Build history of the part. All positions in model axes, mm. Face numbers are marked on the shaded views. A direction names the side the tool comes from. Round coordinates to 2 decimals unless told otherwise and drop trailing zeros. Write each loop counter-clockwise with the first axis right and the second up, starting at its lowest first coordinate (ties: lowest second). Pieces come first, ordered by that corner, then holes. Notation, with made-up numbers: (-22.5, -16) -> (18.5, -16) arc R18 cw to (18.5, 7) -> close; hole circle Ø4 at (-39, -18.75). An arc over 180 degrees is marked (long way). Answer in a Markdown table with one row per item.
```python
from build123d import *

# Parameters (mm, degrees)
BOSS_EXTRUDE1_DEPTH = 5
SKETCH2_R           = 10
BOSS_EXTRUDE2_DEPTH = 10
SKETCH3_R           = 5
CUT_EXTRUDE1_DEPTH  = 10
BOSS_EXTRUDE3_START = 10
SKETCH4_R           = 10
BOSS_EXTRUDE3_DEPTH = 10
BOSS_EXTRUDE4_DEPTH = 5
SKETCH9_R           = 5
CUT_EXTRUDE4_DEPTH  = 35


with BuildPart() as part:
    # Sketch1 → Boss-Extrude1 (new body)
    with BuildSketch(Plane.XY):
        with BuildLine():
            Line((10, 10), (10, 200))
            ThreePointArc((10, 200), (0, 210), (-10, 200))
            Line((-10, 200), (-10, 10))
            ThreePointArc((-10, 10), (0, 0), (10, 10))
        make_face()
    extrude(amount=BOSS_EXTRUDE1_DEPTH)

    # Sketch2 → Boss-Extrude2 (add)
    with BuildSketch(Plane.XY.offset(5)):
        with Locations((0, 200)):
            Circle(SKETCH2_R)
        with Locations((0, 10)):
            Circle(SKETCH2_R)
    extrude(amount=BOSS_EXTRUDE2_DEPTH)

    # Sketch3 → Cut-Extrude1 (cut)
    with BuildSketch(Plane(origin=(0, 0, 0), x_dir=(-1, 0, 0), z_dir=(0, 0, -1))):
        with Locations((0, 105)):
            Circle(SKETCH3_R)
    extrude(amount=-CUT_EXTRUDE1_DEPTH, mode=Mode.SUBTRACT)

    # Sketch4 → Boss-Extrude3 (add)
    with BuildSketch(Plane(origin=(0, 0, 0), x_dir=(-1, 0, 0), z_dir=(0, 0, -1)).offset(BOSS_EXTRUDE3_START)):
        with Locations((0, 200)):
            Circle(SKETCH4_R)
        with Locations((0, 10)):
            Circle(SKETCH4_R)
    extrude(amount=-BOSS_EXTRUDE3_DEPTH)

    # Sketch5 → Boss-Extrude4 (add)
    with BuildSketch(Plane(origin=(0, 0, 0), x_dir=(-1, 0, 0), z_dir=(0, 0, -1))):
        with BuildLine():
            Line((12, 200), (12, 10))
            ThreePointArc((12, 10), (0, -2), (-12, 10))
            Line((-12, 10), (-12, 200))
            ThreePointArc((-12, 200), (0, 212), (12, 200))
        make_face()
    extrude(amount=-BOSS_EXTRUDE4_DEPTH)

    # Sketch9 → Cut-Extrude4 (cut)
    with BuildSketch(Plane(origin=(0, 0, 0), x_dir=(-1, 0, 0), z_dir=(0, 0, -1))):
        with Locations((0, 105)):
            Circle(SKETCH9_R)
    extrude(amount=-CUT_EXTRUDE4_DEPTH, mode=Mode.SUBTRACT)


solid = part.part
```
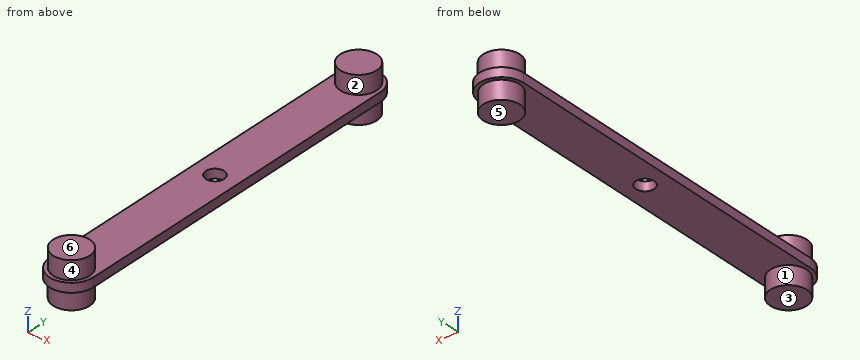
Q1. Wall check: line 1 (Y direction, x = 0, z = 1.35); line 2 (Y direction, x = 1.5, z = 6); line 3 (Z direction, x = -5.5, y = 143.5). Give the ranges that are in metal, low to high. Write a range as [from, to].
A:
| item | result |
|---|---|
| line 1 | [-2, 100], [110, 212] |
| line 2 | [0.11, 19.89], [190.11, 209.89] |
| line 3 | [0, 5] |
Q2. Saw through at A-A on x = 0. Write the cut outline in (y, z).
A:
| item | result |
|---|---|
| outline | (-2, 0) -> (0, 0) -> (0, -10) -> (20, -10) -> (20, 0) -> (100, 0) -> (100, 5) -> (20, 5) -> (20, 15) -> (0, 15) -> (0, 5) -> (-2, 5) -> close; (110, 0) -> (190, 0) -> (190, -10) -> (210, -10) -> (210, 0) -> (212, 0) -> (212, 5) -> (210, 5) -> (210, 15) -> (190, 15) -> (190, 5) -> (110, 5) -> close |
Q3. Saw through at B-B on y = 105. Write the cut outline in (x, z).
A:
| item | result |
|---|---|
| outline | (-12, 0) -> (-5, 0) -> (-5, 5) -> (-12, 5) -> close; (5, 0) -> (12, 0) -> (12, 5) -> (5, 5) -> close |
Q4. Drop flat-ended pins along their axis: P1, Ø2, axis at x = -7, z = -0.5, coming from the +Y side; P2, Ø12, axis at x = -8, z = -2.5, coming from the +Y side; P3, Ø1, axis at x = 9.5, y = 35, coming from the -Z side; P4, Ø8, axis at x = 0, y = 105, coming from the -Z side. Give the stop position or say it passes through.
A:
| item | result |
|---|---|
| P1 | y = 210.31 |
| P2 | y = 211.73 |
| P3 | z = 0 |
| P4 | through |
Q5. Two-plate mould, pull along Z, no slides. Class the marked faces 4, 5 and 6: released by +Z, released by -Z, zero draft, split by the parting line, or undercut.
A:
| item | result |
|---|---|
| face 4 | zero draft |
| face 5 | released by -Z |
| face 6 | released by +Z |
Q6. Which spindle directions (+Z, -Z, +X, -X, +Y, -Y) get a long thin tool onto all of the face, cutting with end or side? Do the marked faces 1, 2 and 3. Say none if no direction does.
A:
| item | result |
|---|---|
| face 1 | -Z |
| face 2 | +Z |
| face 3 | -Z, +X, -X, +Y, -Y |
Q7. Saw through at C-C on y = 52. Write the cut outline in (x, z).
A:
| item | result |
|---|---|
| outline | (-12, 0) -> (12, 0) -> (12, 5) -> (-12, 5) -> close |
